```python
from build123d import *

# Parameters (mm, degrees)
EXTRUDE_THIN1_DEPTH = 1828.8
EXTRUDE_THIN3_DEPTH = 1828.8


with BuildPart() as part:
    # Sketch1 → Extrude-Thin1 (new body)
    with BuildSketch(Plane(origin=(0, 0, 0), x_dir=(1, 0, 0), z_dir=(0, 1, 0))):
        with BuildLine():
            Line((-863.6, 152.4), (863.6, 152.4))
            ThreePointArc((863.6, 152.4), (899.521024484, 137.521024484), (914.4, 101.6))
            Line((914.4, 101.6), (914.4, -101.6))
            ThreePointArc((914.4, -101.6), (899.521024484, -137.521024484), (863.6, -152.4))
            Line((863.6, -152.4), (-863.6, -152.4))
            ThreePointArc((-863.6, -152.4), (-899.521024484, -137.521024484), (-914.4, -101.6))
            Line((-914.4, -101.6), (-914.4, 101.6))
            ThreePointArc((-914.4, 101.6), (-899.521024484, 137.521024484), (-863.6, 152.4))
        make_face()
        with BuildLine():
            Line((-863.6, 130.175), (863.6, 130.175))
            ThreePointArc((863.6, 130.175), (883.805576272, 121.805576272), (892.175, 101.6))
            Line((892.175, 101.6), (892.175, -101.6))
            ThreePointArc((892.175, -101.6), (883.805576272, -121.805576272), (863.6, -130.175))
            Line((863.6, -130.175), (-863.6, -130.175))
            ThreePointArc((-863.6, -130.175), (-883.805576272, -121.805576272), (-892.175, -101.6))
            Line((-892.175, -101.6), (-892.175, 101.6))
            ThreePointArc((-892.175, 101.6), (-883.805576272, 121.805576272), (-863.6, 130.175))
        make_face(mode=Mode.SUBTRACT)
    extrude(amount=EXTRUDE_THIN1_DEPTH)

    # Sketch2 → Extrude-Thin3 (add)
    with BuildSketch(Plane(origin=(0, 1828.8, 0), x_dir=(1, 0, 0), z_dir=(0, 1, 0))):
        Polygon((-879.97255462, -132.236089264), (-201.982109296, 116.912927618), (0, -148.525916816), (201.982109296, 116.912927618), (879.97255462, -132.236089264), (887.638597925, -111.375063281), (194.237534197, 143.437072382), (0, -111.824083184), (-194.237534197, 143.437072382), (-887.638597925, -111.375063281), align=None)
    extrude(amount=-EXTRUDE_THIN3_DEPTH)


solid = part.part
```
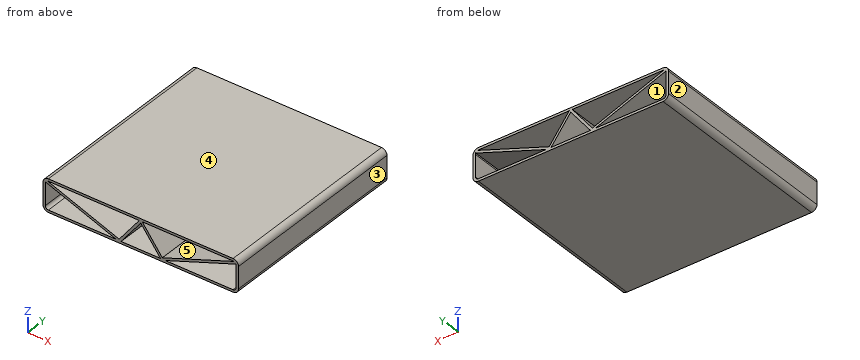
The model under review builds one solid part; all positions refer to its coordinate system, in mm. Face numbers are marked on the shaded views. A direction names the side the tool comes from. Round coordinates to 2 decimals unless told otherwise and drop trailing zeros. Loops run counter-clockwise (first coordinate to the right, second up) from the corner with the lowest first, then second, coordinate; pieces in that order, holes last. Notation, with made-up numbers: (-16.75, -3) - (32.25, -3) arc R13 ccw to (32.25, 5) - close; hole circle Ø9 at (51, -29). An arc over 180 degrees is marked (long way). Use a Markdown table: item, result. Add a question column.
Q1. Add section A-A (z = 6). State the section outline as (x, y) points (3 decimals), plus the area to 3 significant figures.
Q2. For probe 1 along Z at (x, y) = (156, 492) (3 decimals); probe 2 along Z at (x, y) = (-316, 1670) (3 decimals); probe 3 along Z at (x, y) = (225, 1365.5) (3 decimals), list the stretches that pass through material, from the lowest coordinate up.
Q3. Add section C-C (x = 668.5). State the section outline as (y, z) points (3 decimals), plus the area to 3 significant figures.
Q4. Add section B-B (y = 1369.5). State how many separate pieces and enclosed holes the cut face has, plus the area to 3 significant figures.
Q5. The part is to be moulded in two halves that separate along X. For the marked faces 1, 2 and 3, say which applies: pulls with the +X half, pulls with the -X half, needs draft (parallel to the pull), parting line crosses it, or undercut.
Q6. Insertion check: pin 1 Ø1.5 at (y, z) = (1335.5, 110.5) entering from +X. The pin has a flat end and moves straight along its axis. Give the tip position at first contact, or say it passes through.
Q7. Machinability: for the marked faces 4 and 5, which of the approach directions +Z, -Z, +X, -X, +Y, -Y give a long, thin tool a straight path to every point of the face, cutting with its end or side? Answer none if there is none.
Worked answers:
| question | item | result |
|---|---|---|
| 1 | outline | (-914.4, 0) - (-892.175, 0) - (-892.175, 1828.8) - (-914.4, 1828.8) - close; (-600.889, 0) - (-536.456, 0) - (-536.456, 1828.8) - (-600.889, 1828.8) - close; (-108.453, 0) - (-80.525, 0) - (-80.525, 1828.8) - (-108.453, 1828.8) - close; (80.525, 0) - (108.453, 0) - (108.453, 1828.8) - (80.525, 1828.8) - close; (536.456, 0) - (600.889, 0) - (600.889, 1828.8) - (536.456, 1828.8) - close; (892.175, 0) - (914.4, 0) - (914.4, 1828.8) - (892.175, 1828.8) - close |
| 1 | area | 419,000 mm² |
| 2 | probe 1 | -152.4 to -130.175, -93.186 to -56.485, 130.175 to 152.4 |
| 2 | probe 2 | -152.4 to -130.175, -98.692 to -75.013, 130.175 to 152.4 |
| 2 | probe 3 | -152.4 to -108.454, 130.175 to 152.4 |
| 3 | outline | (0, -152.4) - (1828.8, -152.4) - (1828.8, -130.175) - (0, -130.175) - close; (0, 30.846) - (1828.8, 30.846) - (1828.8, 54.524) - (0, 54.524) - close; (0, 130.175) - (1828.8, 130.175) - (1828.8, 152.4) - (0, 152.4) - close |
| 3 | area | 125,000 mm² |
| 4 | separate pieces | 1 |
| 4 | enclosed holes | 5 |
| 4 | area | 137,000 mm² |
| 5 | face 1 | undercut |
| 5 | face 2 | pulls with the -X half |
| 5 | face 3 | pulls with the +X half |
| 6 | pin 1 | x = 913.74 |
| 7 | face 4 | +Z, +X, -X, +Y, -Y |
| 7 | face 5 | +Y, -Y |
